Autodesk Inventor part; units mm, degrees
ref_plane "YZ Plane" through (0, 0, 0) normal (1, 0, 0) x (0, 1, 0)
ref_plane "XZ Plane" through (0, 0, 0) normal (0, 1, 0) x (-1, 0, 0)
ref_plane "XY Plane" through (0, 0, 0) normal (0, 0, 1) x (1, 0, 0)
sketch "Skizze1" plane through (0, 0, 0) normal (1, 0, 0) x (0, 1, 0)
  line L0 (-23, 20) -> (23, 20)
  line L1 (23, 20) -> (23, -20)
  line L2 (23, -20) -> (-23, -20)
  line L3 (-23, -20) -> (-23, 20)
  line L4 (-23, 20) -> (23, -20) construction
  line L5 (23, 20) -> (-23, -20) construction
  point P0 (0, 0)
  dimension "d0" = 46
  dimension "d1" = 40
extrude "Extrusion1" add sketch "Skizze1" along normal blind 50
sketch "Skizze2" plane through (0, -23, 20) normal (0, 0, 1) x (1, 0, 0)
  line L0 (0, 0) -> (0, 46)
  line L1 (0, 0) -> (50, 0)
  line L2 (50, 46) -> (50, 0)
  line L3 (0, 46) -> (50, 46)
  line L4 (50, 46) -> (50, 0)
  line L5 (50, 40.5) -> (6, 40.5)
  line L6 (6, 40.5) -> (6, 5.5)
  line L7 (6, 5.5) -> (50, 5.5)
  line L8 (50, 5.5) -> (50, 40.5)
  point P0 (0, 23)
  dimension "d4" = 5.5
  dimension "d5" = 5.5
  dimension "d6" = 6
extrude "Extrusion2" cut sketch "Skizze2" against normal through all contours L7 L6 L5 L2
sketch "Skizze3" plane through (0, -23, -20) normal (0, -1, 0) x (1, 0, 0)
  line L0 (0, 0) -> (0, 40)
  line L1 (0, 0) -> (50, 0)
  line L2 (50, 40) -> (50, 0)
  line L3 (0, 40) -> (50, 40)
  line L4 (0, 20) -> (44.7617, 20) construction
  line L5 (20, 34.75) -> (50, 34.75)
  line L6 (50, 34.75) -> (50, 5.25)
  line L7 (50, 5.25) -> (20, 5.25)
  line L8 (20, 5.25) -> (20, 34.75)
  line L9 (20, 34.75) -> (50, 5.25) construction
  line L10 (50, 34.75) -> (20, 5.25) construction
  point P0 (35, 20)
  dimension "d9" = 29.5
  dimension "d10" = 30
extrude "Extrusion3" cut sketch "Skizze3" against normal through all contours L7 L8 L5 L2
sketch "Skizze4" plane through (0, -23, -20) normal (0, -1, 0) x (1, 0, 0)
  line L0 (50, 5.25) -> (20, 5.25)
  line L1 (20, 5.25) -> (20, 34.75)
  line L2 (20, 34.75) -> (50, 34.75)
  line L3 (50, 40) -> (50, 34.75)
  line L4 (0, 40) -> (50, 40)
  line L5 (0, 0) -> (0, 40)
  line L6 (0, 0) -> (50, 0)
  line L7 (50, 5.25) -> (50, 0)
  line L8 (0, 20) -> (84.4351, 20) construction
  point P0 (25, 37.3)
  point P1 (25, 2.7)
  point P2 (17.2, 31)
  point P3 (17.2, 9)
  point P4 (47, 37.3)
  point P5 (47, 2.7)
  dimension "d13" = 5
  dimension "d14" = 5
  dimension "d15" = 34.6
  dimension "d16" = 17.3
  dimension "d17" = 22
  dimension "d18" = 11
  dimension "d19" = 2.8
  dimension "d20" = 2.8
  dimension "d47" = 17.3
  dimension "d48" = 17.3
  dimension "d49" = 22
  dimension "d50" = 22
hole "Bohrung1" at (25, -23, 17.3) at (25, -23, -17.3) at (17.2, -23, 11) at (17.2, -23, -11) at (47, -23, 17.3) at (47, -23, -17.3) direction (0, 1, 0) diameter 2.9 end through all
sketch "Skizze7" plane through (6, -17.5, 20) normal (1, 0, 0) x (0, 0, -1)
  line L0 (29, 8.5) -> (11, 8.5)
  line L1 (11, 8.5) -> (11, 26.5)
  line L2 (11, 26.5) -> (29, 26.5)
  line L3 (29, 26.5) -> (29, 8.5)
  line L4 (29, 8.5) -> (11, 26.5) construction
  line L5 (11, 8.5) -> (29, 26.5) construction
  point P0 (20, 17.5)
  dimension "d52" = 18
  dimension "d53" = 18
hole "Bohrung3" at (6, -9, 9) at (6, 9, 9) at (6, 9, -9) at (6, -9, -9) direction (-1, 0, 0) diameter 3.4 end through all
equation "\"d5\" = d4"
equation "\"d53\" = d52"
properties part number "connection_hand" material "Aluminium 6061"
Verification items for the finished model (mm, model axes). A direction names the side the tool comes from. Coordinates: 2 decimals unless noted, no trailing zeros. Loops run counter-clockwise (first coordinate to the right, second up) from the corner with the lowest first, then second, coordinate; pieces in that order, holes last. Notation, with made-up numbers: (89, -8) -> (95, -8) arc R20 cw to (95, 11) -> close; hole circle Ø7 at (49.5, 33.25). An arc over 180 degrees is marked (long way). Answer as a JSON object with one key per item and string values. Group by question number.
Item 1: Sectioned sample at D-D on x = 21.5. Record the boundary of the cut face in (y, z), plus the area to 4 significant figures.
Item 2: Mould release check, pull along Z, two halves, no side actions. Record for faces 1 (the flat face through (5, 2, -20)), 2 (the cylindrical face through (48.286, -20.212, -17.969)), 3 (the cylindrical face through (17.14, -20.21, 12.45)), 4 (the flat face through (50, 20, 17)): +Z half, -Z half, draft (parallel to the pull), parting line (faces both ways), or undercut.
Item 3: Sectioned sample at A-A on x = 47. State how many separate pieces and enclosed holes the cut face has, plus the area to 3 significant figures.
Item 4: Sectioned sample at C-C on z = 17.3. Record the boundary of the cut face in (x, y), plus the area to 3 significant figures.
Item 5: Tool access check on faces 5 (the cylindrical face through (48.416, 20.288, 17.614)), 6 (the flat face through (35, -20, 14.75)), 7 (the flat face through (18, -17.5, 0)). Record the directions out of +Z, -Z, +X, -X, +Y, -Y that give a thin tool (end or side, any length) a straight path to the whole face; none if there is none.
Item 6: Depth check by flat-ended pin: pin 1 (1.5 mm diameter, centred on y = 6, z = 7, fed in from +X); pin 2 (3 mm diameter, centred on y = 20, z = 3.5, fed in from +X); pin 3 (12 mm diameter, centred on x = 45, y = 6.5, fed in from -Z). Enter the tip coordinate at first touch or a pass-through.
Item 7: Scan lines: probe 1 along Z at (x, y) = (17, 19); probe 2 along Y at (x, z) = (17, -1); probe 3 along X at (y, z) = (20, -17.3). Record each from-to range of solid material in increasing order.
Item 8: Sectioned sample at B-B on y = -9. Record the boundary of the cut face in (x, z), plus the area to 3 significant figures.
Evaluation:
{
 "1": {"outline": "(-23, -20) -> (-17.5, -20) -> (-17.5, -14.75) -> (-23, -14.75) -> close; (-23, 14.75) -> (-17.5, 14.75) -> (-17.5, 20) -> (-23, 20) -> close; (17.5, -20) -> (23, -20) -> (23, -14.75) -> (17.5, -14.75) -> close; (17.5, 14.75) -> (23, 14.75) -> (23, 20) -> (17.5, 20) -> close", "area": "115.5 mm²"},
 "2": {"face 1": "-Z half", "face 2": "undercut", "face 3": "undercut", "face 4": "draft"},
 "3": {"separate pieces": "8", "enclosed holes": "0", "area": "51.7 mm²"},
 "4": {"outline": "(0, -23) -> (23.55, -23) -> (23.55, -17.5) -> (6, -17.5) -> (6, 17.5) -> (23.55, 17.5) -> (23.55, 23) -> (0, 23) -> close; (26.45, -23) -> (45.55, -23) -> (45.55, -17.5) -> (26.45, -17.5) -> close; (26.45, 17.5) -> (45.55, 17.5) -> (45.55, 23) -> (26.45, 23) -> close; (48.45, -23) -> (50, -23) -> (50, -17.5) -> (48.45, -17.5) -> close; (48.45, 17.5) -> (50, 17.5) -> (50, 23) -> (48.45, 23) -> close", "area": "696 mm²"},
 "5": {"face 5": "+Y, -Y", "face 6": "+X, +Y, -Y", "face 7": "+Z, -Z, +X"},
 "6": {"pin 1": "stops at x = 6", "pin 2": "stops at x = 20", "pin 3": "passes through"},
 "7": {"probe 1": "z = -20 to -12.44, -9.56 to 9.56, 12.44 to 20", "probe 2": "y = -23 to -17.5, 17.5 to 23", "probe 3": "x = 0 to 23.55, 26.45 to 45.55, 48.45 to 50"},
 "8": {"outline": "(0, -20) -> (6, -20) -> (6, -10.7) -> (0, -10.7) -> close; (0, -7.3) -> (6, -7.3) -> (6, 7.3) -> (0, 7.3) -> close; (0, 10.7) -> (6, 10.7) -> (6, 20) -> (0, 20) -> close", "area": "199 mm²"}
}
